Print and shaded views of the part. All mm, measured from the part's lowest x, y and z. A direction names the side the tool comes from. Give positions to 0.01 mm unless a question says otherwise; leave off trailing zeros. Write each loop counter-clockwise with the first axis right and the second up, starting at its lowest first coordinate (ties: lowest second). Pieces come first, ordered by that corner, then holes.
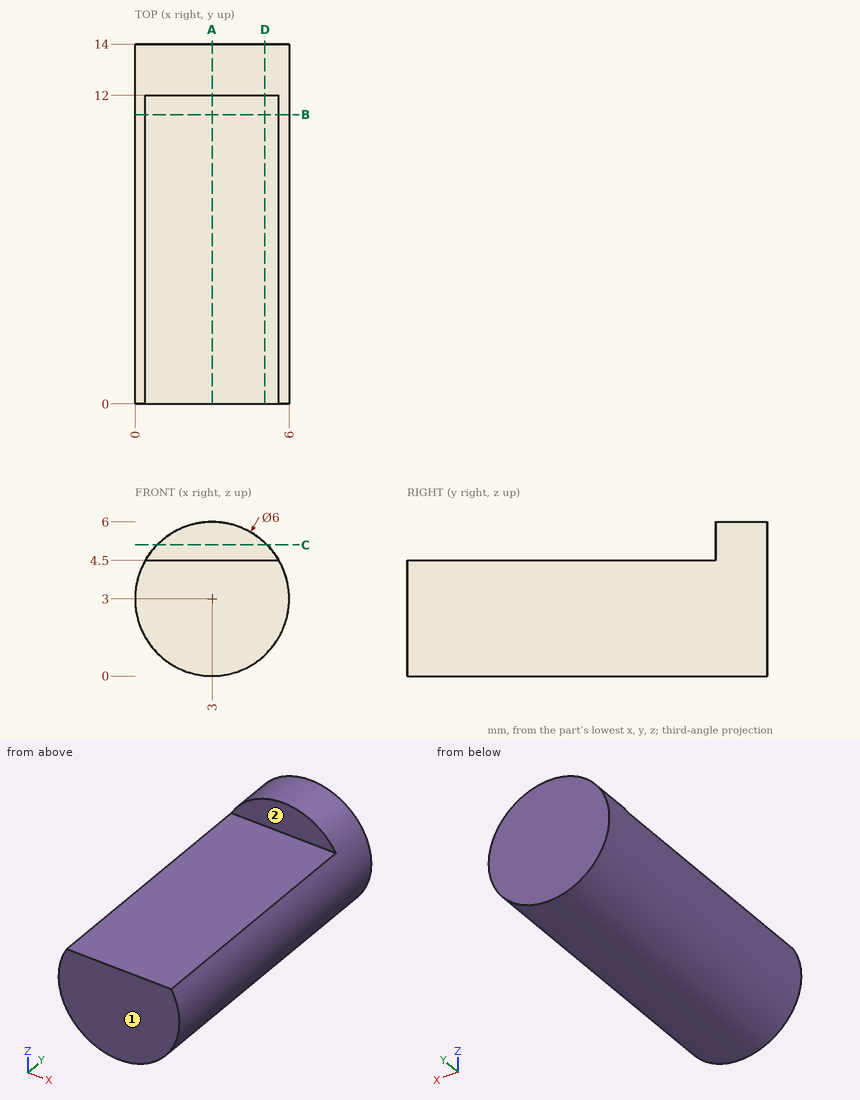
1. 3-axis set-ups, long thin cutter, end or side, ignore diameter. For the marked faces 1 and 2: which of +Z, -Z, +X, -X, +Y, -Y reach the whole face in a straight line?
2. Saw through at B-B on y = 11.25. Give the cut face in (x, z), plus the area to 3 significant figures.
3. Saw through at A-A on x = 3. Give the cut face in (y, z), plus the area to 3 significant figures.
4. Drop flat-ended pins along their axis: pin 1 (3 mm diameter, centred on x = 4, y = 10, fed in from +Z); pin 2 (3 mm diameter, centred on x = 1.5, z = 5, fed in from -Y). Give the stop position or say it passes through.
5. Drill centre lines: line 1 along X through (y, z) = (6, 3.5); line 2 along X through (y, z) = (2.5, 0.55); line 3 along Z through (x, y) = (1, 3). Where is each one in solid material? Low to high.
6. Saw through at C-C on z = 5.1. Give the cut face in (x, y), plus the area to 3 significant figures.
7. Saw through at D-D on x = 5.05. Give the cut face in (y, z).
Outcome:
1. face 1: +Z, -Z, +X, -X, -Y
1. face 2: +Z, +X, -X, -Y
2. outline: (0.4, 4.5) arc R3 ccw (long way) to (5.6, 4.5) - close
2. area: 22.7 mm2
3. outline: (0, 0) - (14, 0) - (14, 6) - (12, 6) - (12, 4.5) - (0, 4.5) - close
3. area: 66.0 mm2
4. pin 1: stops at z = 4.5
4. pin 2: stops at y = 0
5. line 1: x = 0.04 to 5.96
5. line 2: x = 1.27 to 4.73
5. line 3: z = 0.76 to 4.5
6. outline: (0.86, 12) - (5.14, 12) - (5.14, 14) - (0.86, 14) - close
6. area: 8.57 mm2
7. outline: (0, 0.81) - (14, 0.81) - (14, 5.19) - (12, 5.19) - (12, 4.5) - (0, 4.5) - close
